Could you check a few things on this model? Use its own coordinates, in mm. A direction names the side the tool comes from. Round coordinates to 2 decimals unless told otherwise and drop trailing zeros. Loops run counter-clockwise (first coordinate to the right, second up) from the corner with the lowest first, then second, coordinate; pieces in that order, holes last. Notation, with made-up numbers: (-1, 75.25) -> (48, 75.25) arc R14 cw to (48, 88.25) -> close; hole circle Ø2 at (21, 22). An arc over 180 degrees is marked (long way). One line per item, written item: value.
from build123d import *

# Parameters (mm, degrees)
SKETCH2_R           = 2
BOSS_EXTRUDE1_DEPTH = 3
SKETCH6_R           = 3.5
SKETCH6_R_2         = 2
BOSS_EXTRUDE2_DEPTH = 2
FILLET1_R           = 0.5
FILLET4_R           = 0.5


with BuildPart() as part:
    # Sketch2 → Boss-Extrude1 (new body)
    with BuildSketch(Plane(origin=(0, 0, 0), x_dir=(1, 0, 0), z_dir=(0, 1, 0))):
        Polygon((4.041451884, 0), (2.020725942, 3.5), (-2.020725942, 3.5), (-4.041451884, 0), (-2.020725942, -3.5), (2.020725942, -3.5), align=None)
        with Locations(Location((0, 0, 0), (0, 0, 270))):
            Circle(SKETCH2_R, mode=Mode.SUBTRACT)
    extrude(amount=BOSS_EXTRUDE1_DEPTH)

    # Sketch6 → Boss-Extrude2 (add)
    with BuildSketch(Plane(origin=(0, 3, 0), x_dir=(1, 0, 0), z_dir=(0, 1, 0))):
        with Locations(Location((0, 0, 0), (0, 0, 270))):
            Circle(SKETCH6_R)
        with Locations(Location((0, 0, 0), (0, 0, 270))):
            Circle(SKETCH6_R_2, mode=Mode.SUBTRACT)
    extrude(amount=BOSS_EXTRUDE2_DEPTH)

    # Fillet1
    fillet1_edges = [part.edges().sort_by_distance(p)[0] for p in [
        (0, 5, -3.5),
    ]]
    fillet(fillet1_edges, radius=FILLET1_R)

    # Fillet4
    fillet4_edges = [part.edges().sort_by_distance(p)[0] for p in [
        (2.020725942, 1.5, 3.5),
        (-2.020725942, 1.5, 3.5),
        (-4.041451884, 1.5, 0),
        (-2.020725942, 1.5, -3.5),
        (2.020725942, 1.5, -3.5),
        (4.041451884, 1.5, 0),
    ]]
    fillet(fillet4_edges, radius=FILLET4_R)


solid = part.part
(1) Thinking about a two-plate mould opening in Z: for faces 1 (the face through (-1.86, 3, -3.15)), 2 (the face through (3.043, 1.479, -1.729)), 3 (the face through (-2, 2, 0)), 4 (the face through (0, 1, 3.5)), which applies, released by +Z, released by -Z, zero draft, split by the parting line, or undercut?
Recorded:
face 1: zero draft
face 2: released by -Z
face 3: undercut
face 4: released by +Z
(2) If we section it at B-B, the plane y = 2.5: Please give me the cut outline in (x, z).
Recorded:
outline: (-3.9, -0.25) -> (-2.17, -3.25) arc R0.5 ccw to (-1.73, -3.5) -> (1.73, -3.5) arc R0.5 ccw to (2.17, -3.25) -> (3.9, -0.25) arc R0.5 ccw to (3.9, 0.25) -> (2.17, 3.25) arc R0.5 ccw to (1.73, 3.5) -> (-1.73, 3.5) arc R0.5 ccw to (-2.17, 3.25) -> (-3.9, 0.25) arc R0.5 ccw to start; hole circle Ø4 at (0, 0)
(3) I'm going to push a flat-ended pin straight in: pin 1 Ø1.9 at (x, z) = (2, -2.5) entering from +Y. Where does the tip first touch, or does it pass through?
Recorded:
pin 1: y = 5
(4) For faces 5 (the face through (-1.9, 3, 3.2)), 6 (the face through (-3.417, 3.74, -0.759)), 7 (the face through (3.7, 3, 0)), 8 (the face through (1.85, 3, -3.15)), 9 (the face through (1.8, 3, 3.2)), which set-ups out of +Z, -Z, +X, -X, +Y, -Y let a thin tool reach every point of the face, with its end or its side?
Recorded:
face 5: +Z, -X, +Y
face 6: +Y
face 7: +X, +Y
face 8: -Z, +X, +Y
face 9: +Z, +X, +Y
(5) If I drill on L1, parallel to X at y = 2.5, z = 0; L2, parallel to X at y = 3.4, z = 0; L3, parallel to X at y = 2.8, z = 3.25, over which ranges is the centre line in solid material (lowest first)?
Recorded:
L1: -3.96 to -2, 2 to 3.96
L2: -3.5 to -2, 2 to 3.5
L3: -2.17 to 2.17
(6) If we section it at A-A, the plane z = 0: Please give me the cut outline in (x, y), then the cut area to 3 significant figures.
Recorded:
outline: (-3.96, 0) -> (-2, 0) -> (-2, 5) -> (-3, 5) arc R0.5 ccw to (-3.5, 4.5) -> (-3.5, 3) -> (-3.96, 3) -> close; (2, 0) -> (3.96, 0) -> (3.96, 3) -> (3.5, 3) -> (3.5, 4.5) arc R0.5 ccw to (3, 5) -> (2, 5) -> close
area: 17.7 mm²
